Model file for the job. Use its own axes, mm. Give positions to 0.01 mm unless a question says otherwise; leave off trailing zeros. Loops run counter-clockwise (first coordinate to the right, second up) from the corner with the lowest first, then second, coordinate; pieces in that order, holes last. Notation, with made-up numbers: (81.25, 26.5) - (95.25, 26.5) arc R33 cw to (95.25, 57.5) - close; hole circle Ø10 at (-26.75, 87.5). An arc over 180 degrees is marked (long way). Use a Markdown table: item, result.
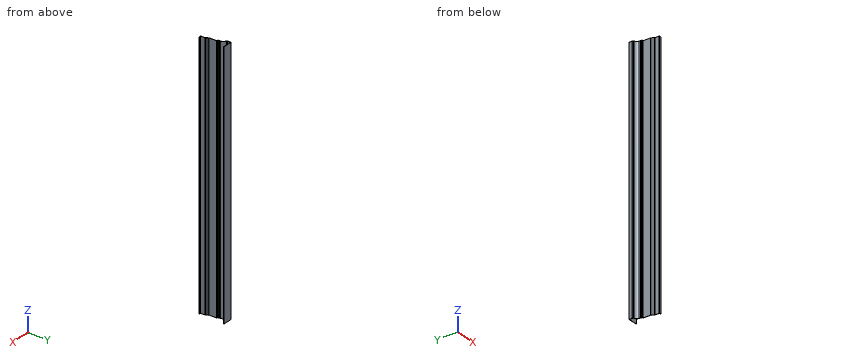
from build123d import *

# Parameters (mm, degrees)
EXTRUDE_THIN1_DEPTH = 1095.375
FILLET1_R           = 1.016


with BuildPart() as part:
    # Sketch1 → Extrude-Thin1 (new body)
    with BuildSketch(Plane.XY):
        with BuildLine():
            Line((0, 0), (-8.73125, 0))
            Line((-8.73125, 0), (-8.73125, 19.05))
            Line((-8.73125, 19.05), (-10.31875, 19.05))
            ThreePointArc((-10.31875, 19.05), (-10.936141439, 22.255855924), (-12.7, 25.003125))
            ThreePointArc((-12.7, 25.003125), (-14.463858561, 27.750394076), (-15.08125, 30.95625))
            Line((-15.08125, 30.95625), (-16.66875, 30.95625))
            Line((-16.66875, 30.95625), (-16.66875, 64.29375))
            Line((-16.66875, 64.29375), (-19.690990213, 64.29375))
            ThreePointArc((-19.690990213, 64.29375), (-22.556015121, 64.295224921), (-22.148203112, 67.131077398))
            Line((-22.148203112, 67.131077398), (-20.250068746, 68.351516354))
            ThreePointArc((-20.250068746, 68.351516354), (-19.937393927, 69.05810986), (-20.463483992, 69.624033147))
            Line((-20.463483992, 69.624033147), (-23.01875, 70.246875))
            Line((-23.01875, 70.246875), (-23.01875, 76.596875))
            ThreePointArc((-23.01875, 76.596875), (-26.970977871, 86.138397129), (-36.5125, 90.090625))
            Line((-36.5125, 90.090625), (-36.5125, 94.45625))
            Line((-36.5125, 94.45625), (-38.1, 94.45625))
            Line((-38.1, 94.45625), (-38.1, 109.5375))
            Line((-38.1, 109.5375), (1.5875, 109.5375))
            Line((1.5875, 109.5375), (1.5875, 108.5215))
            Line((1.5875, 108.5215), (-37.084, 108.5215))
            Line((-37.084, 108.5215), (-37.084, 95.47225))
            Line((-37.084, 95.47225), (-35.4965, 95.47225))
            Line((-35.4965, 95.47225), (-35.4965, 91.071010175))
            ThreePointArc((-35.4965, 91.071010175), (-25.899424313, 86.491088942), (-22.00275, 76.596875))
            Line((-22.00275, 76.596875), (-22.00275, 71.044973159))
            Line((-22.00275, 71.044973159), (-20.222880084, 70.611132818))
            ThreePointArc((-20.222880084, 70.611132818), (-18.935387932, 69.226157431), (-19.700592224, 67.496921976))
            Line((-19.700592224, 67.496921976), (-21.59872659, 66.27648302))
            ThreePointArc((-21.59872659, 66.27648302), (-21.64120221, 64.825375438), (-20.272663327, 65.30975))
            Line((-20.272663327, 65.30975), (-15.65275, 65.30975))
            Line((-15.65275, 65.30975), (-15.65275, 31.97225))
            Line((-15.65275, 31.97225), (-13.99717715, 31.97225))
            ThreePointArc((-13.99717715, 31.97225), (-13.693796997, 28.60677814), (-11.964275862, 25.703814655))
            ThreePointArc((-11.964275862, 25.703814655), (-10.194199045, 23.100527755), (-9.356394818, 20.066))
            Line((-9.356394818, 20.066), (-7.71525, 20.066))
            Line((-7.71525, 20.066), (-7.71525, 1.016))
            Line((-7.71525, 1.016), (0, 1.016))
            Line((0, 1.016), (0, 0))
        make_face()
    extrude(amount=-EXTRUDE_THIN1_DEPTH)

    # Fillet1
    fillet1_edges = [part.edges().sort_by_distance(p)[0] for p in [
        (-35.4965, 95.47225, -547.6875),
        (-20.272663327, 65.30975, -547.6875),
        (-15.65275, 65.30975, -547.6875),
        (-13.99717715, 31.97225, -547.6875),
        (-7.71525, 20.066, -547.6875),
        (-8.73125, 0, -547.6875),
        (-10.31875, 19.05, -547.6875),
        (-16.66875, 30.95625, -547.6875),
        (-23.01875, 70.246875, -547.6875),
        (-36.5125, 90.090625, -547.6875),
        (-38.1, 94.45625, -547.6875),
        (-38.1, 109.5375, -547.6875),
    ]]
    fillet(fillet1_edges, radius=FILLET1_R)


solid = part.part
(1) Slice it at A-A, the plane y = 52.5. Write the cut outline in (x, z) (3 decimals).
Computed:
| item | result |
|---|---|
| outline | (-16.669, -1095.375) - (-15.653, -1095.375) - (-15.653, 0) - (-16.669, 0) - close |
(2) Pin check, flat tips, straight feed: P1, Ø2.5, axis at x = -18.5, z = -347, coming from the -Y side; P2, Ø1, axis at y = 68.5, z = -714, coming from the -X side; P3, Ø1.1, axis at y = 0.5, z = -741.5, coming from the +X side; P4, Ø11.5, axis at x = -9, z = -481, coming from the -Y side. Stop position of each tip, or through.
Computed:
| item | result |
|---|---|
| P1 | y = 64.23 |
| P2 | x = -20.8 |
| P3 | x = 0 |
| P4 | y = 0 |
(3) Drill centre lines: probe 1 along Y at (x, z) = (-16, -584); probe 2 along Y at (x, z) = (-2, -683); probe 3 along Y at (x, z) = (0.5, -54.5). Where is each one in solid material? Low to high. Write a range as [from, to].
Computed:
| item | result |
|---|---|
| probe 1 | [31.02, 65.06], [108.52, 109.54] |
| probe 2 | [0, 1.02], [108.52, 109.54] |
| probe 3 | [108.52, 109.54] |
